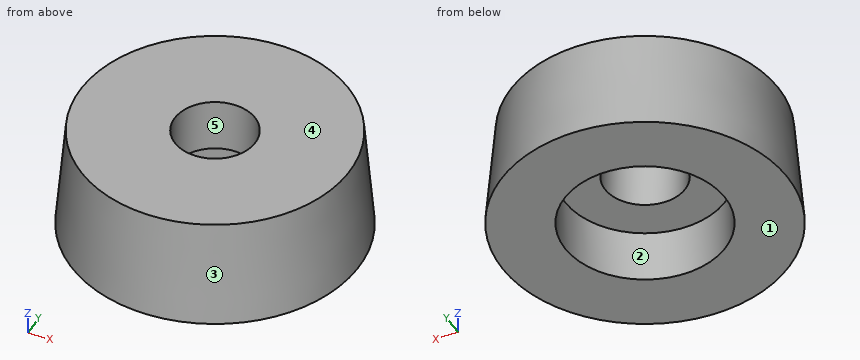
from build123d import *

# Parameters (mm, degrees)
SKETCH_1_R          = 10
SKETCH_1_R_2        = 3
EXTRUDE_1_DEPTH     = 8
DRAFT_1_ANGLE       = 5
SKETCH_2_R          = 6
CUT_EXTRUDE_1_DEPTH = 4


with BuildPart() as part:
    # 草图1 → 凸台-拉伸1 (new body)
    with BuildSketch(Plane.XY):
        Circle(SKETCH_1_R)
        Circle(SKETCH_1_R_2, mode=Mode.SUBTRACT)
    extrude(amount=EXTRUDE_1_DEPTH)

    # 拔模1
    draft_1_faces = [part.faces().sort_by_distance(p)[0] for p in [
        (-10, 0, 4),
    ]]
    draft(draft_1_faces, Plane.XY.offset(8), DRAFT_1_ANGLE)

    # 草图2 → 切除-拉伸1 (cut)
    with BuildSketch(Plane(origin=(0, 0, 0), x_dir=(-1, 0, 0), z_dir=(0, 0, -1))):
        Circle(SKETCH_2_R)
    extrude(amount=-CUT_EXTRUDE_1_DEPTH, mode=Mode.SUBTRACT)


solid = part.part
Work out the finished part from the listing and answer in its coordinate system (mm). Face numbers are marked on the shaded views. A direction names the side the tool comes from. Give positions to 0.01 mm unless a question says otherwise; leave off trailing zeros. Write each loop counter-clockwise with the first axis right and the second up, starting at its lowest first coordinate (ties: lowest second). Pieces come first, ordered by that corner, then holes.
Q1. The part is cut by section D-D on z = 3. Give the vertices of the cut face in (x, y).
Answer:
outline: circle Ø20.87 at (0, 0); hole circle Ø12 at (0, 0)
Q2. Given pin 1 (3 mm diameter, centred on y = -4.5, z = 6, fed in from +X); pin 2 (2 mm diameter, centred on x = 8.5, z = 1, fed in from -Y); pin 3 (2 mm diameter, centred on x = -1, y = -2, fed in from -Z); pin 4 (5.5 mm diameter, centred on x = 0, y = 0, fed in from +Z), each flat-ended and moving along its own axis, determine where each tip first touches the part or whether it passes through.
Answer:
pin 1: stops at x = 9.74
pin 2: stops at y = -7.52
pin 3: stops at z = 4
pin 4: passes through
Q3. Straight lines are drawn through the part: L1, parallel to Z at x = 2, y = -4.75; L2, parallel to Y at x = 0, z = 0.9; L3, parallel to X at y = 2.5, z = 7.5. For each, find the intervals that lie inside material, in ascending order.
Answer:
L1: z = 4 to 8
L2: y = -10.62 to -6, 6 to 10.62
L3: x = -9.73 to -1.66, 1.66 to 9.73
Q4. The part is cut by section A-A on x = 0. Give the vertices of the cut face in (y, z), and give its area (3 significant figures).
Answer:
outline: (-10.7, 0) - (-6, 0) - (-6, 4) - (-3, 4) - (-3, 8) - (-10, 8) - close; (3, 4) - (6, 4) - (6, 0) - (10.7, 0) - (10, 8) - (3, 8) - close
area: 93.6 mm2
Q5. For a pull along Y with two mould halves and no side action, classify the marked faces 3, 4 and 5 as released by +Y, released by -Y, zero draft, split by the parting line, or undercut.
Answer:
face 3: split by the parting line
face 4: zero draft
face 5: undercut
Q6. A tool of negligible diameter and unlimited length cuts with its end or side. For the marked faces 1 and 2, from which of +Z, -Z, +X, -X, +Y, -Y can it reach the whole face along a straight path? Write none if from no direction.
Answer:
face 1: -Z, +X, -X, +Y, -Y
face 2: -Z
Q7. The part is cut by section C-C on z = 5.75. Give the vertices of the cut face in (x, y).
Answer:
outline: circle Ø20.39 at (0, 0); hole circle Ø6 at (0, 0)
